```python
from build123d import *

# Parameters (mm, degrees)
BOSS_EXTRUDE1_DEPTH                               = 100
CSK_FOR_4_FLAT_HEAD_MACHINE_SCREW_100_D           = 3.2639
CSK_FOR_4_FLAT_HEAD_MACHINE_SCREW_100_CSINK_D     = 5.715
CSK_FOR_4_FLAT_HEAD_MACHINE_SCREW_100_CSINK_ANGLE = 100
CSK_FOR_4_FLAT_HEAD_MACHINE_SCREW_2_D             = 3.2639
CSK_FOR_4_FLAT_HEAD_MACHINE_SCREW_2_CSINK_D       = 5.715
CSK_FOR_4_FLAT_HEAD_MACHINE_SCREW_2_CSINK_ANGLE   = 100
FILLET1_R                                         = 1
CSK_FOR_4_FLAT_HEAD_MACHINE_SCREW_3_D             = 3.2639
CSK_FOR_4_FLAT_HEAD_MACHINE_SCREW_3_CSINK_D       = 5.715
CSK_FOR_4_FLAT_HEAD_MACHINE_SCREW_3_CSINK_ANGLE   = 100
CSK_FOR_4_FLAT_HEAD_MACHINE_SCREW_4_D             = 3.2639
CSK_FOR_4_FLAT_HEAD_MACHINE_SCREW_4_CSINK_D       = 5.715
CSK_FOR_4_FLAT_HEAD_MACHINE_SCREW_4_CSINK_ANGLE   = 100
CUT_EXTRUDE1_DEPTH                                = 25


with BuildPart() as part:
    # Sketch2 → Boss-Extrude1 (new, symmetric)
    with BuildSketch(Plane.XY):
        with BuildLine():
            Line((-9.525, 0), (9.525, 0))
            Line((9.525, 0), (9.525, 19.05))
            Line((9.525, 19.05), (8.73125, 19.05))
            ThreePointArc((8.73125, 19.05), (8.169983992, 18.817516008), (7.9375, 18.25625))
            Line((7.9375, 18.25625), (7.9375, 2.38125))
            ThreePointArc((7.9375, 2.38125), (7.705016008, 1.819983992), (7.14375, 1.5875))
            Line((7.14375, 1.5875), (-8.73125, 1.5875))
            ThreePointArc((-8.73125, 1.5875), (-9.292516008, 1.355016008), (-9.525, 0.79375))
            Line((-9.525, 0.79375), (-9.525, 0))
        make_face()
    extrude(amount=BOSS_EXTRUDE1_DEPTH, both=True)

    # CSK for _4 Flat Head Machine Screw _100 (through all)
    with Locations(Plane(origin=(0, 0, 0), x_dir=(-1, 0, 0), z_dir=(0, -1, 0))):
        with Locations((-1.185, -96), (-0.275, 96)):
            CounterSinkHole(CSK_FOR_4_FLAT_HEAD_MACHINE_SCREW_100_D / 2, CSK_FOR_4_FLAT_HEAD_MACHINE_SCREW_100_CSINK_D / 2, counter_sink_angle=CSK_FOR_4_FLAT_HEAD_MACHINE_SCREW_100_CSINK_ANGLE)

    # CSK for _4 Flat Head Machine Screw _ 2 (through all)
    with Locations(Plane(origin=(9.525, 0, 0), x_dir=(0, 0, -1), z_dir=(1, 0, 0))):
        with Locations((-96, 13.5875), (96, 13.5875)):
            CounterSinkHole(CSK_FOR_4_FLAT_HEAD_MACHINE_SCREW_2_D / 2, CSK_FOR_4_FLAT_HEAD_MACHINE_SCREW_2_CSINK_D / 2, counter_sink_angle=CSK_FOR_4_FLAT_HEAD_MACHINE_SCREW_2_CSINK_ANGLE)

    # Fillet1
    fillet1_edges = [part.edges().sort_by_distance(p)[0] for p in [
        (9.525, 0, 0),
    ]]
    fillet(fillet1_edges, radius=FILLET1_R)

    # CSK for _4 Flat Head Machine Screw _ 3 (through all)
    with Locations(Plane(origin=(0, 0, 0), x_dir=(-1, 0, 0), z_dir=(0, -1, 0))):
        with Locations((-0.275, 0)):
            CounterSinkHole(CSK_FOR_4_FLAT_HEAD_MACHINE_SCREW_3_D / 2, CSK_FOR_4_FLAT_HEAD_MACHINE_SCREW_3_CSINK_D / 2, counter_sink_angle=CSK_FOR_4_FLAT_HEAD_MACHINE_SCREW_3_CSINK_ANGLE)

    # CSK for _4 Flat Head Machine Screw _ 4 (through all)
    with Locations(Plane(origin=(9.525, 0, 0), x_dir=(0, 0, -1), z_dir=(1, 0, 0))):
        with Locations((0, 13.5875)):
            CounterSinkHole(CSK_FOR_4_FLAT_HEAD_MACHINE_SCREW_4_D / 2, CSK_FOR_4_FLAT_HEAD_MACHINE_SCREW_4_CSINK_D / 2, counter_sink_angle=CSK_FOR_4_FLAT_HEAD_MACHINE_SCREW_4_CSINK_ANGLE)

    # Sketch26 → Cut-Extrude1 (cut)
    with BuildSketch(Plane.XY.offset(100)):
        Polygon((2.9375, 1.5875), (7.9375, 1.5875), (7.9375, 6.5875), align=None)
    cut_extrude1 = extrude(amount=-CUT_EXTRUDE1_DEPTH, mode=Mode.SUBTRACT)

    # Mirror1: Cut-Extrude1 across plane
    add(cut_extrude1.mirror(Plane.XY), mode=Mode.SUBTRACT)


solid = part.part
```
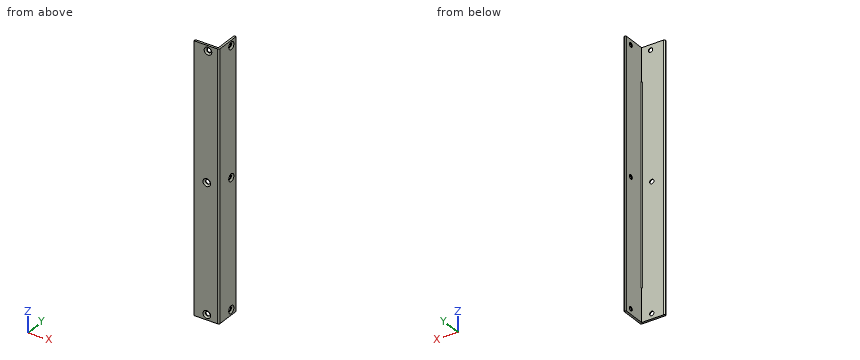
Geometry: final body of the model. Coordinates: model frame, mm. Round coordinates to 2 decimals unless told otherwise and drop trailing zeros. Order: outer loops, then holes, each group sorted by start corner. A loop starts at its lowest first (then second) coordinate and runs counter-clockwise, first axis right, second up. Notation, with made-up numbers: M 20.5,22.5 L 44.5,22.5 A22 cw 44.5,40.5 Z; hole C 86.25,78 d9. An arc over 180 degrees is marked long. One line per item, written item: value.
(1) Pin query (flat end, axial travel): P1, Ø5, axis at x = 0.275, z = 0, coming from the -Y side; P2, Ø8.5, axis at y = 11.5, z = -2.5, coming from the -X side; P3, Ø4, axis at y = 13.59, z = 96, coming from the +X side. Return the tip coordinate at first contact, or that it passes through.
Result sheet:
P1: y = 0.3
P2: x = 7.94
P3: x = 8.81
(2) Cut plane D-D (y = 6.5). Return the cut outline in (x, z) (1 decimal), and give its area (4 significant figures).
Result sheet:
outline: M 7.9,-100 L 9.5,-100 L 9.5,100 L 7.9,100 Z
area: 317.5 mm2
(3) Line query: probe 1 along X at (y, z) = (7.25, -41) (1 decimal); probe 2 along Y at (x, z) = (3.5, 53); probe 3 along Y at (x, z) = (8.4, 96). Output: solid intervals per line, ascending. Write a range as [from, to].
Result sheet:
probe 1: [7.9, 9.5]
probe 2: [0, 1.59]
probe 3: [0, 11.96], [15.22, 18.98]
(4) Cut plane C-C (x = -4.5). Return the cut outline in (y, z).
Result sheet:
outline: M 0,-100 L 1.59,-100 L 1.59,100 L 0,100 Z
(5) Cut plane A-A (z = 96). Give the number of separate pieces and of enclosed holes in the cut face, and give its area (3 significant figures).
Result sheet:
separate pieces: 3
enclosed holes: 0
area: 44.6 mm2
